Geometry: final body of the model. Coordinates: model frame, mm. Round coordinates to 2 decimals unless told otherwise and drop trailing zeros. Loops run counter-clockwise (first coordinate to the right, second up) from the corner with the lowest first, then second, coordinate; pieces in that order, holes last. Notation, with made-up numbers: (3.25, 0.5) - (30.25, 0.5) arc R18 ccw to (30.25, 8.5) - close; hole circle Ø5 at (-2.5, 4.5). An arc over 180 degrees is marked (long way). Write item = value, one per line. Start each with the question number.
Item 1: Section A-A (y = 32). Return loops of the section in (x, z).
Item 2: First-contact query: pin 1 (2 mm diameter, centred on y = 37.5, z = -1.5, fed in from +X) (3 decimals). Flat tip, straight axial feed; report the tip coordinate or a pass-through.
Item 3: Line query: line 1 (X direction, y = 10, z = 0.15); line 2 (Z direction, x = 0.2, y = 35.5); line 3 (Z direction, x = 1.95, y = 30.5). Output: solid intervals per line, ascending. Write a range as from..to.
from build123d import *

# Parameters (mm, degrees)
SKETCH1_R           = 4
BOSS_EXTRUDE1_DEPTH = 50
FILLET1_R           = 1
FILLET2_R           = 1
SCALE1_SCALE        = 0.7


with BuildPart() as part:
    # Sketch1 → Boss-Extrude1 (new body)
    with BuildSketch(Plane(origin=(0, 0, 0), x_dir=(1, 0, 0), z_dir=(0, 1, 0))):
        with Locations(Location((0, 0, 0), (0, 0, 270))):
            Circle(SKETCH1_R)
    extrude(amount=BOSS_EXTRUDE1_DEPTH)

    # Fillet1
    fillet1_edges = [part.edges().sort_by_distance(p)[0] for p in [
        (0, 50, -4),
    ]]
    fillet(fillet1_edges, radius=FILLET1_R)

    # Fillet2
    fillet2_edges = [part.edges().sort_by_distance(p)[0] for p in [
        (0, 0, -4),
    ]]
    fillet(fillet2_edges, radius=FILLET2_R)


with BuildPart() as part_1:
    # Scale1: scaled about (0, 25, 0)
    add(part.part.scale(SCALE1_SCALE).moved(Location((0, 7.5, 0))))


solid = part_1.part
Taken from the geometry:
q1.outline = circle Ø5.6 at (0, 0)
q2.pin_1 = 2.755
q3.line_1 = -2.8..2.8
q3.line_2 = -2.79..2.79
q3.line_3 = -2.01..2.01
